```python
from build123d import *

# Parameters (mm, degrees)
F1_DEPTH = 71
F3_DEPTH = 16
F4_DEPTH = 6
F5_W     = 25.042631
F5_H     = 12
F6_DEPTH = 12.4


with BuildPart() as f1:
    # F0 (on Front) → F1 (new body, symmetric)
    with BuildSketch(Plane.XZ):
        with BuildLine():
            Line((25, -3), (25, 8))
            Line((25, 8), (-25, 8))
            Line((-25, 8), (-25, -8))
            Line((-25, -8), (20, -8))
            ThreePointArc((20, -8), (21.464466, -4.464466), (25, -3))
        make_face()
    extrude(amount=F1_DEPTH, both=True)

    # F2 (on face) → F3 (cut)
    with BuildSketch(Plane.XY.offset(8)):
        with BuildLine():
            ThreePointArc((0, -6), (4.242641, -4.242641), (6, 0))
            ThreePointArc((6, 0), (4.242641, 4.242641), (0, 6))
            ThreePointArc((0, 6), (-6, 0), (0, -6))
        make_face()
    extrude(amount=-F3_DEPTH, mode=Mode.SUBTRACT)

    # F2 (on face) → F4 (cut)
    with BuildSketch(Plane.XY.offset(8)):
        with BuildLine():
            ThreePointArc((0, 6), (4.242641, 4.242641), (6, 0))
            ThreePointArc((6, 0), (4.242641, -4.242641), (0, -6))
            Line((0, -6), (25, -6))
            Line((25, -6), (25, 6))
            Line((25, 6), (0, 6))
        make_face()
    extrude(amount=-F4_DEPTH, mode=Mode.SUBTRACT)

    # F5 (on face) → F6 (cut)
    with BuildSketch(Plane(origin=(0, 0, -8), x_dir=(1, 0, 0), z_dir=(0, 0, -1))):
        with Locations((12.521316, 0)):
            Rectangle(F5_W, F5_H)
    extrude(amount=-F6_DEPTH, mode=Mode.SUBTRACT)


solid = f1.part
```
CAD build for the part. Positions are in the model's coordinates, mm. A direction names the side the tool comes from. Round coordinates to 2 decimals unless told otherwise and drop trailing zeros. Loops run counter-clockwise (first coordinate to the right, second up) from the corner with the lowest first, then second, coordinate; pieces in that order, holes last. Notation, with made-up numbers: M 2.25,-26 L 7.25,-26 A17 ccw 7.25,-5 Z; hole C 61,42 d8. An arc over 180 degrees is marked long. Use a Markdown table: item, result. Add a question column.
(1) Cut at B-B (z = 5.25). Give the cut face in (x, y), and give its area (3 significant figures).
(2) Flat gauge pin, fed straight in: pin 1 (8 mm diameter, centred on y = -54.5, z = -5.5, fed in from +X). Where does the tip first touch, or does it go through?
(3) Cut at A-A (x = 18). Give the cut face in (y, z), and give its area (3 significant figures).
(4) Drill centre lines: line 1 (Y direction, x = 13, z = 3); line 2 (Y direction, x = -4.5, z = -1.5); line 3 (X direction, y = -28.5, z = -4.75). Where is each one in solid material? Low to high.
(5) Which spindle directions (+Z, -Z, +X, -X, +Y, -Y) get a long thin tool onto all of the face, cutting with end or side? Do faces 1 (the face through (-11, -1, 8)), 2 (the face through (13, 6, 0)). Say none if no direction does.
(6) Cut at D-D (z = -5). Give the cut face in (x, y).
(7) Cut at C-C (y = 55). Give the cut face in (x, z), and give its area (3 significant figures).
(8) Pull direction Y, two halves, no side cores. Call faces 3 (the face through (21, 38, -5)), 4 (the face through (12, -6, 0)), 5 (the face through (0, -71, 0)), 6 (the face through (0, 71, 0)): +Y half, -Y half, draft (parallel to the pull), parting line (faces both ways), or undercut.
Geometry says:
| question | item | result |
|---|---|---|
| 1 | outline | M -25,-71 L 25,-71 L 25,-6 L 0,-6 A6 cw 0,6 L 25,6 L 25,71 L -25,71 Z |
| 1 | area | 6,740 mm² |
| 2 | pin 1 | stops at x = 25 |
| 3 | outline | M -71,-8 L -6,-8 L -6,8 L -71,8 Z; M 6,-8 L 71,-8 L 71,8 L 6,8 Z |
| 3 | area | 2,080 mm² |
| 4 | line 1 | y = -71 to -6, 6 to 71 |
| 4 | line 2 | y = -71 to -3.97, 3.97 to 71 |
| 4 | line 3 | x = -25 to 21.2 |
| 5 | face 1 | +Z, +X, -X, +Y, -Y |
| 5 | face 2 | +Z, -Z, +X |
| 6 | outline | M -25,-71 L 21,-71 L 21,-6 L 0,-6 A6 cw 0,6 L 21,6 L 21,71 L -25,71 Z |
| 7 | outline | M -25,-8 L 20,-8 A5 cw 25,-3 L 25,8 L -25,8 Z |
| 7 | area | 780 mm² |
| 8 | face 3 | draft |
| 8 | face 4 | undercut |
| 8 | face 5 | -Y half |
| 8 | face 6 | +Y half |
